from build123d import *

# Parameters (mm, degrees)
F0_W     = 40
F0_H     = 30
F1_DEPTH = 20
F2_T     = -1.2
F4_D     = 25


with BuildPart() as f1:
    # F0 (on Top) → F1 (new body)
    with BuildSketch(Plane.XY):
        with Locations((20, -15)):
            Rectangle(F0_W, F0_H)
    extrude(amount=F1_DEPTH)

    # F2
    f2_openings = [f1.faces().sort_by_distance(p)[0] for p in [
        (20, -15, 0),
    ]]
    offset(amount=F2_T, openings=f2_openings)

    # F4 (through all)
    with Locations(Plane.XY.offset(20)):
        with Locations((20, -15)):
            Hole(F4_D / 2)


solid = f1.part
Here's how the part is built. I have some questions about the finished solid (model axes, mm). A direction names the side the tool comes from. Coordinates: 2 decimals unless noted, no trailing zeros. Write each loop counter-clockwise with the first axis right and the second up, starting at its lowest first coordinate (ties: lowest second). Pieces come first, ordered by that corner, then holes.
1) Thinking about a two-plate mould opening in Y: for faces 3 (the face through (20, -1.2, 9)), 4 (the face through (1.2, -15, 9)), 5 (the face through (20, 0, 10)), 6 (the face through (18, -29, 0)), which applies, +Y half, -Y half, draft (parallel to the pull), parting line (faces both ways), or undercut?
Filled in:
face 3: undercut
face 4: undercut
face 5: +Y half
face 6: draft
2) If we section it at B-B (z = 16.25): List the corners of the cut face in (x, y) for me, plus the area to 3 significant figures.
Filled in:
outline: (0, -30) - (40, -30) - (40, 0) - (0, 0) - close; hole (1.2, -28.8) - (38.8, -28.8) - (38.8, -1.2) - (1.2, -1.2) - close
area: 162 mm2
3) If we section it at A-A (x = 20): List the corners of the cut face in (y, z) for me.
Filled in:
outline: (-30, 0) - (-28.8, 0) - (-28.8, 18.8) - (-27.5, 18.8) - (-27.5, 20) - (-30, 20) - close; (-2.5, 18.8) - (-1.2, 18.8) - (-1.2, 0) - (0, 0) - (0, 20) - (-2.5, 20) - close
4) If I drill on line 1 (Y direction, x = 20, z = 19.5); line 2 (X direction, y = -26, z = 10.75); line 3 (Y direction, x = 22, z = 5.25), over which ranges is the centre line in solid material (lowest first)?
Filled in:
line 1: y = -30 to -27.5, -2.5 to 0
line 2: x = 0 to 1.2, 38.8 to 40
line 3: y = -30 to -28.8, -1.2 to 0
5) Which directions (+Z, -Z, +X, -X, +Y, -Y) give clear straight access to the entire face, cutting with the end or side of a thin tool? Please do faces 1 (the face through (11, -6, 18.8)), 2 (the face through (0, -15, 10)).
Filled in:
face 1: -Z
face 2: +Z, -Z, -X, +Y, -Y
6) I'm going to push a flat-ended pin straight in: pin 1 (14 mm diameter, centred on x = 19, y = -11.5, fed in from -Z). Where does the tip first touch, or does it pass through?
Filled in:
pin 1: passes through
7) If we section it at D-D (y = -2): List the corners of the cut face in (x, z) for me.
Filled in:
outline: (0, 0) - (1.2, 0) - (1.2, 18.8) - (38.8, 18.8) - (38.8, 0) - (40, 0) - (40, 20) - (0, 20) - close
8) If we section it at C-C (y = -15): List the corners of the cut face in (x, z) for me.
Filled in:
outline: (0, 0) - (1.2, 0) - (1.2, 18.8) - (7.5, 18.8) - (7.5, 20) - (0, 20) - close; (32.5, 18.8) - (38.8, 18.8) - (38.8, 0) - (40, 0) - (40, 20) - (32.5, 20) - close
